from build123d import *

# Parameters (mm, degrees)
SKETCH2_W           = 230
SKETCH2_H           = 120
BOSS_EXTRUDE1_DEPTH = 38
CUT_EXTRUDE1_DEPTH  = 28
SKETCH4_W           = 160
SKETCH4_H           = 46
CUT_EXTRUDE2_DEPTH  = 261.929109147
SKETCH5_W           = 311.823210218
SKETCH5_H           = 28.846030915
CUT_EXTRUDE3_DEPTH  = 72
SKETCH6_R           = 3
CUT_EXTRUDE4_DEPTH  = 15
SKETCH7_R           = 3
CUT_EXTRUDE5_DEPTH  = 260.563094449
SKETCH8_R           = 2
CUT_EXTRUDE6_DEPTH  = 261.831363145
SKETCH9_R           = 2.5
CUT_EXTRUDE7_DEPTH  = 261.831363145


with BuildPart() as part:
    # Sketch2 → Boss-Extrude1 (new body)
    with BuildSketch(Plane.XY):
        with Locations((115, -60)):
            Rectangle(SKETCH2_W, SKETCH2_H)
    extrude(amount=BOSS_EXTRUDE1_DEPTH)

    # Sketch3 → Cut-Extrude1 (cut)
    with BuildSketch(Plane.XY.offset(38)):
        Polygon((28, -120), (28, -74), (230, -74), (230, 0), (0, 0), (0, -120), align=None)
    extrude(amount=-CUT_EXTRUDE1_DEPTH, mode=Mode.SUBTRACT)

    # Sketch4 → Cut-Extrude2 (cut, through all)
    with BuildSketch(Plane.XY.offset(10)):
        with Locations((150, -23)):
            Rectangle(SKETCH4_W, SKETCH4_H)
    extrude(amount=-CUT_EXTRUDE2_DEPTH, mode=Mode.SUBTRACT)

    # Sketch5 → Cut-Extrude3 (cut)
    with BuildSketch(Plane.XY.offset(38)):
        with Locations((110.708854905, -131.423015458)):
            Rectangle(SKETCH5_W, SKETCH5_H)
    extrude(amount=-CUT_EXTRUDE3_DEPTH, mode=Mode.SUBTRACT)

    # Sketch6 → Cut-Extrude4 (cut)
    with BuildSketch(Plane(origin=(0, -74, 0), x_dir=(1, 0, 0), z_dir=(0, 1, 0))):
        with Locations(Location((128, -24, 0), (0, 0, 270))):
            Circle(SKETCH6_R)
    extrude(amount=-CUT_EXTRUDE4_DEPTH, mode=Mode.SUBTRACT)

    # Sketch7 → Cut-Extrude5 (cut, through all)
    with BuildSketch(Plane.XY.offset(10)):
        with Locations((14, -15)):
            Circle(SKETCH7_R)
        with Locations((14, -102)):
            Circle(SKETCH7_R)
    extrude(amount=-CUT_EXTRUDE5_DEPTH, mode=Mode.SUBTRACT)

    # Sketch8 → Cut-Extrude6 (cut, through all)
    with BuildSketch(Plane(origin=(0, 0, 0), x_dir=(-1, 0, 0), z_dir=(0, 0, -1))):
        with Locations((-55, -10)):
            Circle(SKETCH8_R)
        with Locations((-55, -40)):
            Circle(SKETCH8_R)
        with Locations((-32, -40)):
            Circle(SKETCH8_R)
        with Locations((-32, -10)):
            Circle(SKETCH8_R)
    extrude(amount=-CUT_EXTRUDE6_DEPTH, mode=Mode.SUBTRACT)

    # Sketch9 → Cut-Extrude7 (cut, through all)
    with BuildSketch(Plane(origin=(0, 0, 0), x_dir=(-1, 0, 0), z_dir=(0, 0, -1))):
        with Locations((-16, -25)):
            Circle(SKETCH9_R)
    extrude(amount=-CUT_EXTRUDE7_DEPTH, mode=Mode.SUBTRACT)


solid = part.part
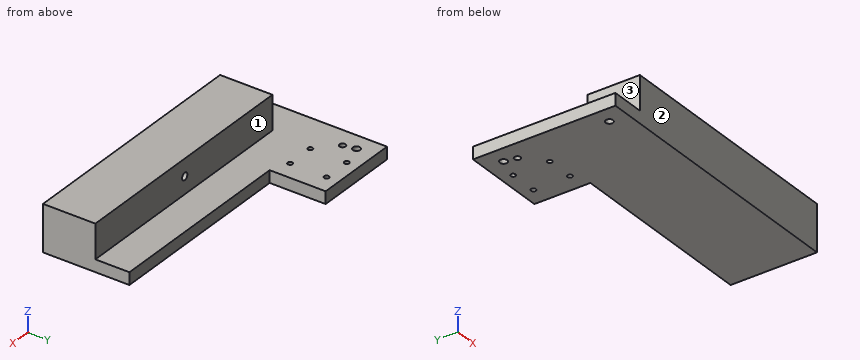
Model file for the job. Use its own axes, mm. Face numbers are marked on the shaded views. A direction names the side the tool comes from. Coordinates: 2 decimals unless noted, no trailing zeros. Write each loop counter-clockwise with the first axis right and the second up, starting at its lowest first coordinate (ties: lowest second). Pieces come first, ordered by that corner, then holes. Notation, with made-up numbers: (30, 43.25) - (71, 43.25) arc R19 ccw to (71, 51.25) - close; hole circle Ø3 at (50.25, -16). An arc over 180 degrees is marked (long way). Write each question's results on one line, items separated by ' | '. Start each with the question number.
1) Cut at B-B (y = -25). Write the cut outline in (x, z), then the cut area to 3 significant figures.
2) Cut at A-A (z = 7). Write the cut outline in (x, y).
3) 3-axis set-ups, long thin cutter, end or side, ignore diameter. For the marked faces 1, 2 and 3: which of +Z, -Z, +X, -X, +Y, -Y reach the whole face in a straight line?
4) Cut at C-C (y = -80). Write the cut outline in (x, z).
5) Flat gauge pins, fed straight in: P1, Ø2, axis at x = 154, z = 4.5, coming from the +Y side; P2, Ø5, axis at x = 129, z = 22.5, coming from the +Y side; P3, Ø12, axis at x = 154, y = -43.5, coming from the +Z side; P4, Ø12, axis at x = 64, y = -50, coming from the -Z side. Where does each tip first touch, or does it go through?
6) Probe line 1 along Y through (x, z) = (32, 5); line 2 along Z through (x, y) = (128, -82); line 3 along Y through (x, z) = (62.5, 11.5). List the from-to ranges inside material, lowest first. Write a range as from..to.
7) Cut at D-D (x = 128). Write the cut outline in (y, z).
Returned:
1) outline: (0, 0) - (13.5, 0) - (13.5, 10) - (0, 10) - close; (18.5, 0) - (70, 0) - (70, 10) - (18.5, 10) - close | area: 650 mm^2
2) outline: (0, -117) - (230, -117) - (230, -46) - (70, -46) - (70, 0) - (0, 0) - close; hole circle Ø6 at (14, -102); hole circle Ø6 at (14, -15); hole circle Ø5 at (16, -25); hole circle Ø4 at (32, -40); hole circle Ø4 at (32, -10); hole circle Ø4 at (55, -40); hole circle Ø4 at (55, -10)
3) face 1: +Z, +X, -X, +Y | face 2: +Z, -Z, +X, -X, -Y | face 3: +Z, -X, +Y, -Y
4) outline: (0, 0) - (230, 0) - (230, 38) - (28, 38) - (28, 10) - (0, 10) - close; hole circle Ø6 at (128, 24)
5) P1: y = -46 | P2: y = -74 | P3: z = 10 | P4: z = 0
6) line 1: -117..-42, -38..-12, -8..0 | line 2: 0..21, 27..38 | line 3: -117..-74
7) outline: (-117, 0) - (-46, 0) - (-46, 10) - (-74, 10) - (-74, 21) - (-89, 21) - (-89, 27) - (-74, 27) - (-74, 38) - (-117, 38) - close
